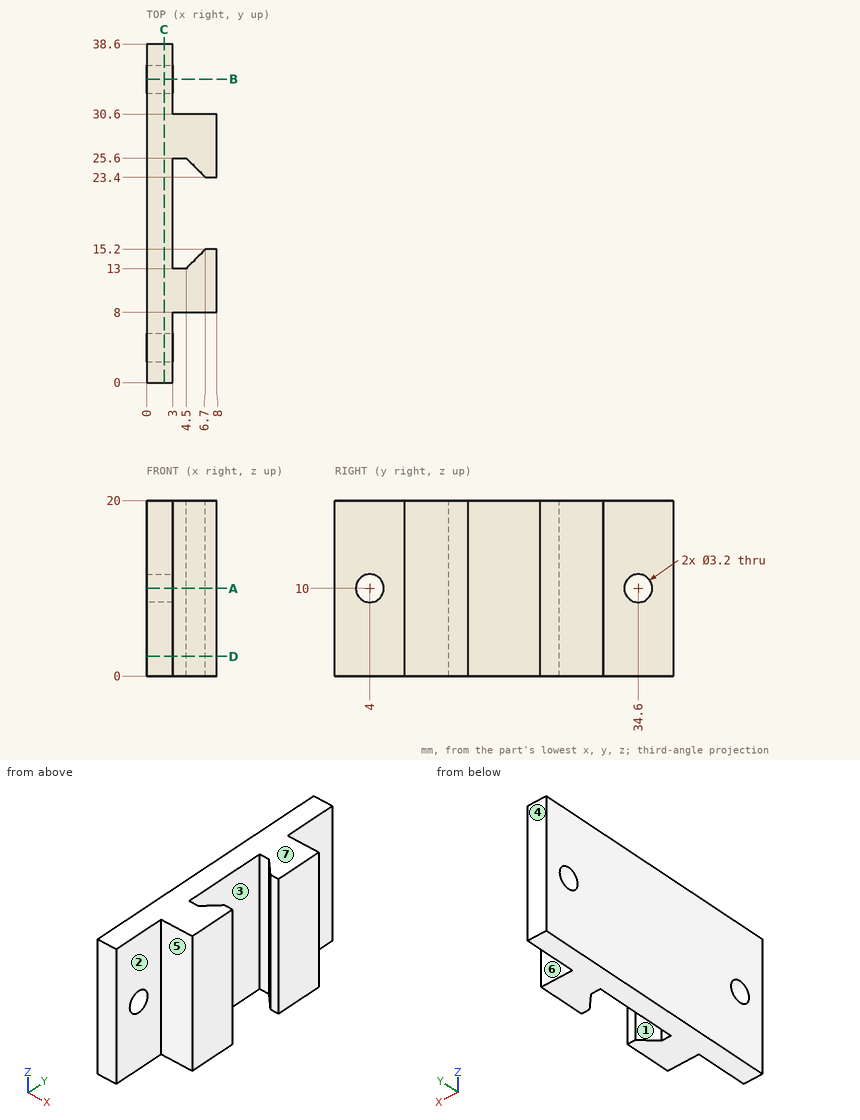
Here's the drawing with two shaded views (mm, measured from the low corner). I have some questions. A direction names the side the tool comes from. Coordinates: 2 decimals unless noted, no trailing zeros. Loops run counter-clockwise (first coordinate to the right, second up) from the corner with the lowest first, then second, coordinate; pieces in that order, holes last. Notation, with made-up numbers: M 26,47.5 L 34,47.5 A16 ccw 34,53.5 Z; hole C -38.5,-24.5 d5. An arc over 180 degrees is marked long. Answer as CSV lines item,"result". Start each with the question number.
1. Suppose I cut it at D-D, the plane z = 2.25. List the corners of the cut face in (x, y) for me, plus the area to 3 significant figures.
2. For pin 1 Ø2.5 at (y, z) = (34.6, 10) entering from -X; pin 2 Ø9 at (y, z) = (4, 7.5) entering from +X; pin 3 Ø1.5 at (x, z) = (5, 10) entering from -Y; pin 4 Ø1 at (x, z) = (7.5, 6) entering from +Y, each with a flat end and sliding along its axis, tell me the tip position at first contact or that it passes through.
3. Thinking about a two-plate mould opening in Y: for the marked faces 1, 2, 3 and 4, which applies, +Y half, -Y half, draft (parallel to the pull), parting line (faces both ways), or undercut?
4. If I drill on probe 1 along Y at (x, z) = (0.65, 10); probe 2 along Y at (x, z) = (7.25, 6.5); probe 3 along Y at (x, z) = (3.5, 16), over which ranges is the centre line in solid material (lowest first)? Write a range as [from, to].
5. For the marked faces 5, 6 and 7, which set-ups out of +Z, -Z, +X, -X, +Y, -Y let a thin tool reach every point of the face, with its end or its side?
6. Suppose I cut it at B-B, the plane y = 34.6. List the corners of the cut face in (x, z) for me, plus the area to 3 significant figures.
7. Suppose I cut it at A-A, the plane z = 10. List the corners of the cut face in (x, y) for me.
8. Suppose I cut it at C-C, the plane x = 2. List the corners of the cut face in (y, z) for me, plus the area to 3 significant figures.
Output:
1,outline,"M 0,0 L 3,0 L 3,8 L 8,8 L 8,15.2 L 6.7,15.2 L 4.5,13 L 3,13 L 3,25.6 L 4.5,25.6 L 6.7,23.4 L 8,23.4 L 8,30.6 L 3,30.6 L 3,38.6 L 0,38.6 Z"
1,area,"176 mm^2"
2,pin 1,"passes through"
2,pin 2,"stops at x = 8"
2,pin 3,"stops at y = 8"
2,pin 4,"stops at y = 30.6"
3,face 1,"undercut"
3,face 2,"draft"
3,face 3,"undercut"
3,face 4,"+Y half"
4,probe 1,"y = [0, 2.4], [5.6, 33], [36.2, 38.6]"
4,probe 2,"y = [8, 15.2], [23.4, 30.6]"
4,probe 3,"y = [8, 13], [25.6, 30.6]"
5,face 5,"+Z, -Z, +X, -Y"
5,face 6,"+Z, -Z, +X, +Y"
5,face 7,"+Z, +X, -X, +Y, -Y"
6,outline,"M 0,0 L 3,0 L 3,8.4 L 0,8.4 Z; M 0,11.6 L 3,11.6 L 3,20 L 0,20 Z"
6,area,"50.4 mm^2"
7,outline,"M 0,0 L 3,0 L 3,2.4 L 0,2.4 Z; M 0,5.6 L 3,5.6 L 3,8 L 8,8 L 8,15.2 L 6.7,15.2 L 4.5,13 L 3,13 L 3,25.6 L 4.5,25.6 L 6.7,23.4 L 8,23.4 L 8,30.6 L 3,30.6 L 3,33 L 0,33 Z; M 0,36.2 L 3,36.2 L 3,38.6 L 0,38.6 Z"
8,outline,"M 0,0 L 38.6,0 L 38.6,20 L 0,20 Z; hole C 4,10 d3.2; hole C 34.6,10 d3.2"
8,area,"756 mm^2"
